Source: three-view drawing plus pictorial views. Frame: mm from the lowest corner of the part. Give positions to 0.01 mm unless a question says otherwise; leave off trailing zeros. Loops run counter-clockwise (first coordinate to the right, second up) from the corner with the lowest first, then second, coordinate; pieces in that order, holes last. Notation, with made-up numbers: M 58.5,48.5 L 96.5,48.5 A20 cw 96.5,75.5 Z; hole C 88.5,48 d3. An arc over 180 degrees is marked long. Answer as a JSON object with one key per item and string values. Group by question number.
1) Ray query, L1, parallel to Z at x = 21.5, y = 1.9; L2, parallel to X at y = 2.3, z = 50.5; L3, parallel to X at y = 0.6, z = 37. Return the intervals inside material, ascending.
2) Section query C-C on z = 68. Return loops of the section in (x, y).
3) Section query B-B on x = 32. Return loops of the section in (y, z).
4) Section query D-D on y = 1. Return loops of the section in (x, z), plus the area to 3 significant figures.
5) First-contact query: P1, Ø0.9, axis at x = 54.5, y = 1.5, coming from the -Z side; P2, Ø0.9, axis at y = 2, z = 55.5, coming from the -X side. Flat tips, straight axial feed; report the tip coordinate or a pass-through.
6) Section query A-A on z = 56.5. Return loops of the section in (x, y), plus the area to 3 significant figures.
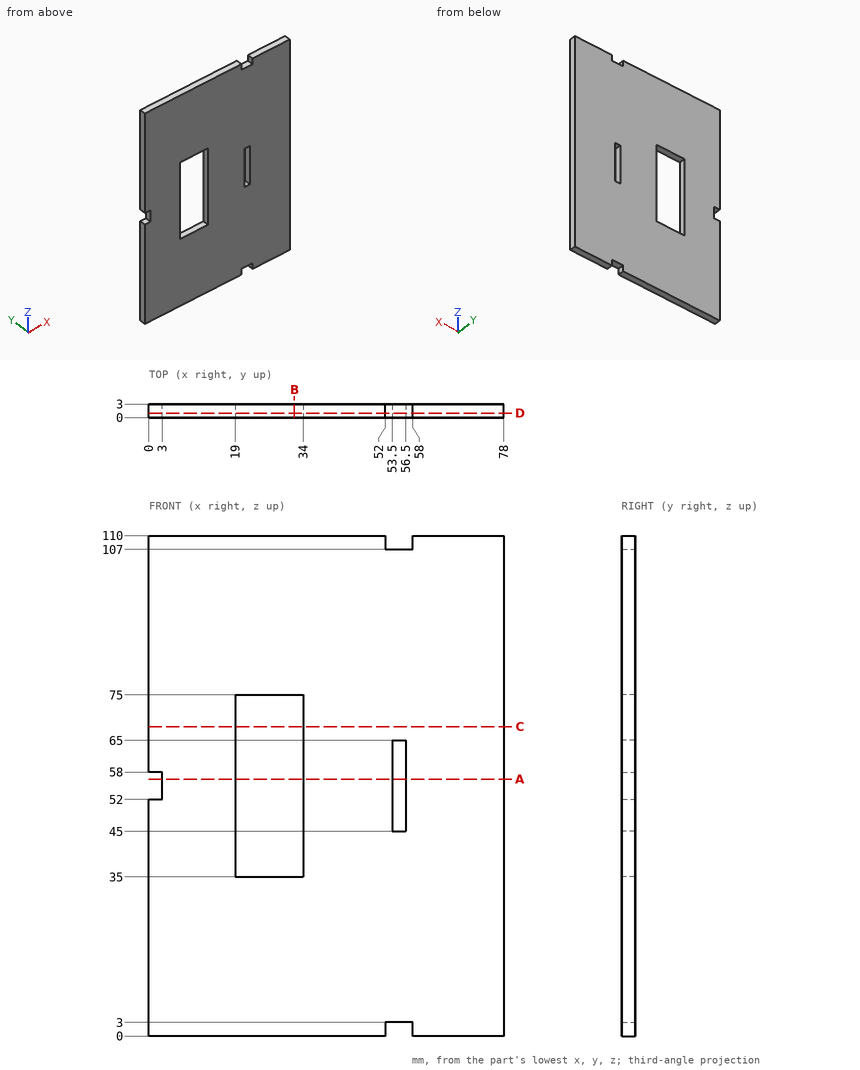
Output:
{
 "1": {"L1": "z = 0 to 35, 75 to 110", "L2": "x = 0 to 19, 34 to 53.5, 56.5 to 78", "L3": "x = 0 to 19, 34 to 78"},
 "2": {"outline": "M 0,0 L 19,0 L 19,3 L 0,3 Z; M 34,0 L 78,0 L 78,3 L 34,3 Z"},
 "3": {"outline": "M 0,0 L 3,0 L 3,35 L 0,35 Z; M 0,75 L 3,75 L 3,110 L 0,110 Z"},
 "4": {"outline": "M 0,0 L 52,0 L 52,3 L 58,3 L 58,0 L 78,0 L 78,110 L 58,110 L 58,107 L 52,107 L 52,110 L 0,110 L 0,58 L 3,58 L 3,52 L 0,52 Z; hole M 19,35 L 34,35 L 34,75 L 19,75 Z; hole M 53.5,45 L 56.5,45 L 56.5,65 L 53.5,65 Z", "area": "7,870 mm^2"},
 "5": {"P1": "stops at z = 3", "P2": "stops at x = 3"},
 "6": {"outline": "M 3,0 L 19,0 L 19,3 L 3,3 Z; M 34,0 L 53.5,0 L 53.5,3 L 34,3 Z; M 56.5,0 L 78,0 L 78,3 L 56.5,3 Z", "area": "171 mm^2"}
}
